Build history of the part. All positions in model axes, mm. Give positions to 0.01 mm unless a question says otherwise; leave off trailing zeros. Order: outer loops, then holes, each group sorted by start corner. A loop starts at its lowest first (then second) coordinate and runs counter-clockwise, first axis right, second up. Notation, with made-up numbers: (-8.75, 20.5) -> (-1.75, 20.5) arc R23 cw to (-1.75, 32.5) -> close; hole circle Ø6 at (79, 62). An arc over 180 degrees is marked (long way). Use a Markdown table: item, result. Add a question column.
```python
from build123d import *

# Parameters (mm, degrees)
SKETCH1_W           = 72
SKETCH1_H           = 46
BOSS_EXTRUDE1_DEPTH = 1.5
BOSS_EXTRUDE2_DEPTH = 1.5
FILLET1_R           = 10
FILLET2_R           = 15
SKETCH4_R           = 2.5
CUT_EXTRUDE1_DEPTH  = 57.751394231
CUT_EXTRUDE2_DEPTH  = 57.751394231


with BuildPart() as part:
    # Sketch1 → Boss-Extrude1 (new body)
    with BuildSketch(Plane(origin=(0, 0, 0), x_dir=(1, 0, 0), z_dir=(0, 1, 0))):
        Rectangle(SKETCH1_W, SKETCH1_H)
    extrude(amount=BOSS_EXTRUDE1_DEPTH)

    # Sketch2 → Boss-Extrude2 (add)
    with BuildSketch(Plane(origin=(0, 0, 0), x_dir=(-1, 0, 0), z_dir=(0, -1, 0))):
        with BuildLine():
            Line((43.855417409, -20.308053614), (27.33033513, -9.129656043))
            Line((27.33033513, -9.129656043), (20.046462909, -19.897441585))
            Line((20.046462909, -19.897441585), (36.571545189, -31.075839157))
            ThreePointArc((36.571545189, -31.075839157), (45.59737407, -29.333882496), (43.855417409, -20.308053614))
        make_face()
        with BuildLine():
            Line((43.855417409, 20.308053614), (27.867856538, 9.493262584))
            Line((27.867856538, 9.493262584), (20.583984318, 20.261048126))
            Line((20.583984318, 20.261048126), (36.571545189, 31.075839157))
            ThreePointArc((36.571545189, 31.075839157), (45.59737407, 29.333882496), (43.855417409, 20.308053614))
        make_face()
        with BuildLine():
            Line((-36.571545189, 31.075839157), (-20.303290898, 20.071172966))
            Line((-20.303290898, 20.071172966), (-27.587163118, 9.303387424))
            Line((-27.587163118, 9.303387424), (-43.855417409, 20.308053614))
            ThreePointArc((-43.855417409, 20.308053614), (-45.59737407, 29.333882496), (-36.571545189, 31.075839157))
        make_face()
        with BuildLine():
            Line((-43.855417409, -20.308053614), (-27.377969487, -9.161878321))
            Line((-27.377969487, -9.161878321), (-20.094097267, -19.929663863))
            Line((-20.094097267, -19.929663863), (-36.571545189, -31.075839157))
            ThreePointArc((-36.571545189, -31.075839157), (-45.59737407, -29.333882496), (-43.855417409, -20.308053614))
        make_face()
    extrude(amount=-BOSS_EXTRUDE2_DEPTH)

    # Fillet1
    fillet1_edges = [part.edges().sort_by_distance(p)[0] for p in [
        (36, 0.75, -14.994253816),
        (36, 0.75, 14.994253816),
        (-36, 0.75, -14.994253816),
        (-36, 0.75, 14.994253816),
    ]]
    fillet(fillet1_edges, radius=FILLET1_R)

    # Fillet2
    fillet2_edges = [part.edges().sort_by_distance(p)[0] for p in [
        (24.632990876, 0.75, -23),
        (24.632990876, 0.75, 23),
        (-24.632990876, 0.75, -23),
        (-24.632990876, 0.75, 23),
    ]]
    fillet(fillet2_edges, radius=FILLET2_R)

    # Sketch4 → Cut-Extrude1 (cut, through all)
    with BuildSketch(Plane(origin=(0, 1.5, 0), x_dir=(1, 0, 0), z_dir=(0, 1, 0))):
        with Locations(Location((-39.954311998, -25.688576308, 0), (0, 0, 270))):
            Circle(SKETCH4_R)
        with Locations(Location((39.954311998, 25.688576308, 0), (0, 0, 270))):
            Circle(SKETCH4_R)
        with Locations(Location((-39.954311998, 25.688576308, 0), (0, 0, 270))):
            Circle(SKETCH4_R)
        with Locations(Location((39.954311998, -25.688576308, 0), (0, 0, 270))):
            Circle(SKETCH4_R)
    extrude(amount=-CUT_EXTRUDE1_DEPTH, mode=Mode.SUBTRACT)

    # Sketch5 → Cut-Extrude2 (cut, through all)
    with BuildSketch(Plane(origin=(0, 1.5, 0), x_dir=(1, 0, 0), z_dir=(0, 1, 0))):
        with BuildLine():
            Line((1.299038106, 6.25), (5.629165125, 13.75))
            ThreePointArc((5.629165125, 13.75), (5.629165125, 15.25), (4.330127019, 16))
            Line((4.330127019, 16), (-4.330127019, 16))
            ThreePointArc((-4.330127019, 16), (-5.629165125, 15.25), (-5.629165125, 13.75))
            Line((-5.629165125, 13.75), (-1.299038106, 6.25))
            ThreePointArc((-1.299038106, 6.25), (0, 5.5), (1.299038106, 6.25))
        make_face()
        with BuildLine():
            Line((-1.299038106, -6.25), (-5.629165125, -13.75))
            ThreePointArc((-5.629165125, -13.75), (-5.629165125, -15.25), (-4.330127019, -16))
            Line((-4.330127019, -16), (4.330127019, -16))
            ThreePointArc((4.330127019, -16), (5.629165125, -15.25), (5.629165125, -13.75))
            Line((5.629165125, -13.75), (1.299038106, -6.25))
            ThreePointArc((1.299038106, -6.25), (0, -5.5), (-1.299038106, -6.25))
        make_face()
        with BuildLine():
            Line((-6.25, 1.299038106), (-13.75, 5.629165125))
            ThreePointArc((-13.75, 5.629165125), (-15.25, 5.629165125), (-16, 4.330127019))
            Line((-16, 4.330127019), (-16, -4.330127019))
            ThreePointArc((-16, -4.330127019), (-15.25, -5.629165125), (-13.75, -5.629165125))
            Line((-13.75, -5.629165125), (-6.25, -1.299038106))
            ThreePointArc((-6.25, -1.299038106), (-5.5, 0), (-6.25, 1.299038106))
        make_face()
        with BuildLine():
            Line((6.25, -1.299038106), (13.75, -5.629165125))
            ThreePointArc((13.75, -5.629165125), (15.25, -5.629165125), (16, -4.330127019))
            Line((16, -4.330127019), (16, 4.330127019))
            ThreePointArc((16, 4.330127019), (15.25, 5.629165125), (13.75, 5.629165125))
            Line((13.75, 5.629165125), (6.25, 1.299038106))
            ThreePointArc((6.25, 1.299038106), (5.5, 0), (6.25, -1.299038106))
        make_face()
    extrude(amount=-CUT_EXTRUDE2_DEPTH, mode=Mode.SUBTRACT)


solid = part.part
```
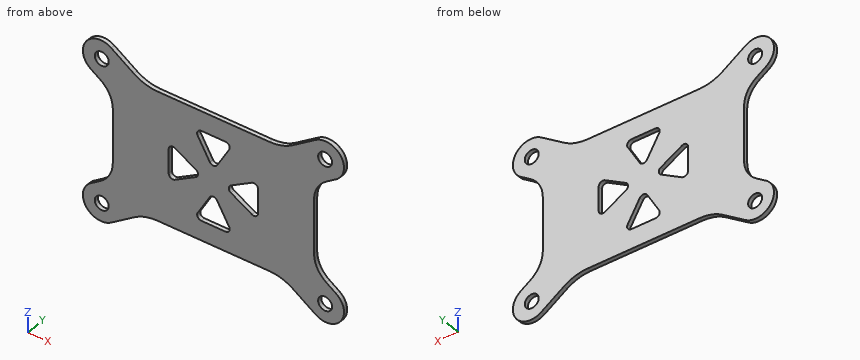
(1) Band-saw the part on A-A on x = 10. Give the cut face in (y, z), plus the area to 3 significant figures.
(2) Pin check, flat tips, straight feed: pin 1 Ø0.8 at (x, y) = (1, 1) entering from +Z; pin 2 Ø0.8 at (x, y) = (-8, 1) entering from -Z; pin 3 Ø0.8 at (y, z) = (1, 1) entering from +X. Stop position of each tip, or through.
(3) Band-saw the part on C-C on x = 23. Give the cut face in (y, z).
(4) Band-saw the part on D-D on y = 0.8. State how many separate pieces and enclosed holes the cut face has, plus the area to 3 significant figures.
(5) Wall check: probe 1 along Z at (x, y) = (38, 1); probe 2 along Z at (x, y) = (-40.5, 1.2); probe 3 along Z at (x, y) = (1, 0.5). Give the ranges that are in metal, low to high.
(6) Band-saw the part on B-B on z = 7.5. Give the cut face in (x, y), plus the area to 3 significant figures.
Response:
| question | item | result |
|---|---|---|
| 1 | outline | (0, -23) -> (1.5, -23) -> (1.5, -3.46) -> (0, -3.46) -> close; (0, 3.46) -> (1.5, 3.46) -> (1.5, 23) -> (0, 23) -> close |
| 1 | area | 58.6 mm² |
| 2 | pin 1 | stops at z = 23 |
| 2 | pin 2 | stops at z = -23 |
| 2 | pin 3 | stops at x = 36 |
| 3 | outline | (0, -23.3) -> (1.5, -23.3) -> (1.5, 23.3) -> (0, 23.3) -> close |
| 4 | separate pieces | 1 |
| 4 | enclosed holes | 8 |
| 4 | area | 3,650 mm² |
| 5 | probe 1 | z = -31.8 to -27.25, -24.13 to -15.69, 15.69 to 24.13, 27.25 to 31.8 |
| 5 | probe 2 | z = -32.19 to -28.13, -23.25 to -18.04, 18.04 to 23.25, 28.13 to 32.19 |
| 5 | probe 3 | z = -23 to -16, -5.88 to 5.88, 16 to 23 |
| 6 | outline | (-36, 0) -> (-2.02, 0) -> (-2.02, 1.5) -> (-36, 1.5) -> close; (2.02, 0) -> (36, 0) -> (36, 1.5) -> (2.02, 1.5) -> close |
| 6 | area | 102 mm² |
